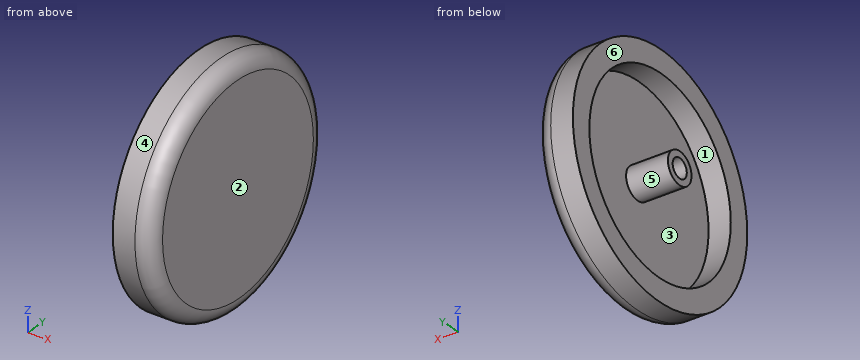
Autodesk Inventor part; units mm, degrees
ref_plane "YZ Plane" through (0, 0, 0) normal (1, 0, 0) x (0, 1, 0)
ref_plane "XZ Plane" through (0, 0, 0) normal (0, 1, 0) x (-1, 0, 0)
ref_plane "XY Plane" through (0, 0, 0) normal (0, 0, 1) x (1, 0, 0)
sketch "Sketch1" plane through (0, 0, 0) normal (1, 0, 0) x (0, 1, 0)
  circle A0 centre (0, 0) radius 23.495
  dimension "d0" = 46.99
extrude "Extrusion1" add sketch "Sketch1" against normal blind 7.62
fillet "Fillet1" radius 3.175 1 edges at (0, -23.495, 0)
sketch "Sketch2" plane through (-7.62, 0, 0) normal (-1, 0, 0) x (0, 0, 1)
  circle A0 centre (0, 0) radius 3.175
  circle A1 centre (0, 0) radius 1.905
  dimension "d4" = 6.35
  dimension "d5" = 3.81
extrude "Extrusion2" add sketch "Sketch2" along normal blind 3.937
sketch "Sketch3" plane through (-7.62, 0, 0) normal (-1, 0, 0) x (0, 0, 1)
  circle A0 centre (0, 0) radius 19.05
  circle A1 centre (0, 0) radius 1.905
  circle A2 centre (0, 0) radius 3.175
  dimension "d8" = 38.1
  dimension "d9" = 6.35
extrude "Extrusion3" cut sketch "Sketch3" against normal blind 4.445 contours A0
properties part number "Chairs Wheel (H)"
For this review, take the finished solid that the model builds, in its own axes (mm). Face numbers are marked on the shaded views. A direction names the side the tool comes from. Coordinates: 2 decimals unless noted, no trailing zeros. Write each loop counter-clockwise with the first axis right and the second up, starting at its lowest first coordinate (ties: lowest second). Pieces come first, ordered by that corner, then holes. Notation, with made-up numbers: (29.5, -23.5) - (55.5, -23.5) arc R20 ccw to (55.5, -9.5) - close; hole circle Ø10 at (70, 29). An arc over 180 degrees is marked (long way). Put each result on its own line as item: value.
1. For pin 1 (1 mm diameter, centred on x = -3.5, y = -16.5, fed in from -Z); pin 2 (4 mm diameter, centred on y = -12.5, z = -2, fed in from -X) (3 decimals); pin 3 (5 mm diameter, centred on x = -10, y = 5, fed in from -Z), all flat-tipped, find the tip position at first contact; note any pin that passes through.
Values found:
pin 1: z = -17.21
pin 2: x = -3.175
pin 3: z = -23.11
2. Mouldability with a two-part tool opening along Z and no side actions: class the marked faces 3, 4, 5 and 6 as released by +Z, released by -Z, zero draft, split by the parting line, or undercut.
Values found:
face 3: undercut
face 4: split by the parting line
face 5: undercut
face 6: zero draft
3. Machinability: for the marked faces 1 and 2, which of the approach directions +Z, -Z, +X, -X, +Y, -Y give a long, thin tool a straight path to every point of the face, cutting with its end or side? Answer none if there is none.
Values found:
face 1: -X
face 2: +Z, -Z, +X, +Y, -Y
4. Wall thickness on probe 1 along Z at (x, y) = (-7.25, 2.5); probe 2 along X at (y, z) = (19, 8); probe 3 along X at (y, z) = (13, -4.5) (3 decimals): over which ranges is each line inside the solid? List them lowest first.
Values found:
probe 1: -23.36 to -18.89, -1.96 to 1.96, 18.89 to 23.36
probe 2: -7.62 to -0.01
probe 3: -3.175 to 0
5. Add section B-B, the plane z = 0. Give the boundary of the cut face in (x, y) (3 decimals), then the cut area to 3 significant figures.
Values found:
outline: (-11.557, -3.175) - (-3.175, -3.175) - (-3.175, -19.05) - (-7.62, -19.05) - (-7.62, -23.495) - (-3.175, -23.495) arc R3.175 ccw to (0, -20.32) - (0, 20.32) arc R3.175 ccw to (-3.175, 23.495) - (-7.62, 23.495) - (-7.62, 19.05) - (-3.175, 19.05) - (-3.175, 3.175) - (-11.557, 3.175) - (-11.557, 1.905) - (-7.62, 1.905) - (-7.62, -1.905) - (-11.557, -1.905) - close
area: 223 mm²
6. Add section A-A, the plane x = -3.75. Give the boundary of the cut face in (y, z) (3 decimals).
Values found:
outline: circle Ø46.99 at (0, 0); circle Ø6.35 at (0, 0); hole circle Ø38.1 at (0, 0)
